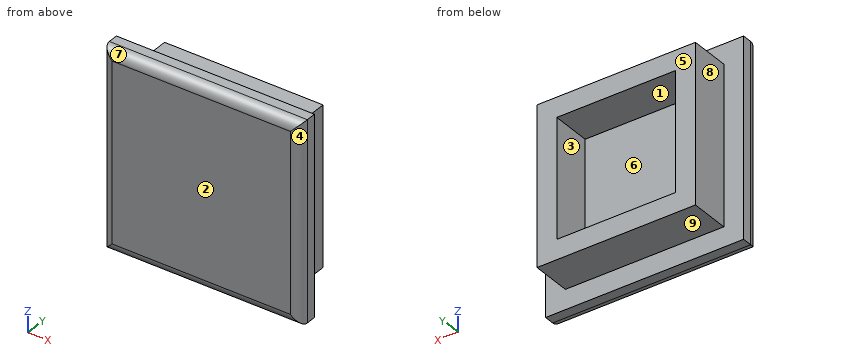
```python
from build123d import *

# Parameters (mm, degrees)
SKETCH1_W           = 20
SKETCH1_H           = 20
BOSS_EXTRUDE1_DEPTH = 2
SKETCH2_W           = 16
SKETCH2_H           = 16
SKETCH2_W_2         = 12
SKETCH2_H_2         = 12
BOSS_EXTRUDE2_DEPTH = 4
FILLET1_R           = 1


with BuildPart() as part:
    # Sketch1 → Boss-Extrude1 (new body)
    with BuildSketch(Plane(origin=(0, 0, 0), x_dir=(1, 0, 0), z_dir=(0, 1, 0))):
        Rectangle(SKETCH1_W, SKETCH1_H)
    extrude(amount=BOSS_EXTRUDE1_DEPTH)

    # Sketch2 → Boss-Extrude2 (add)
    with BuildSketch(Plane(origin=(0, 2, 0), x_dir=(1, 0, 0), z_dir=(0, 1, 0))):
        Rectangle(SKETCH2_W, SKETCH2_H)
        Rectangle(SKETCH2_W_2, SKETCH2_H_2, mode=Mode.SUBTRACT)
    extrude(amount=BOSS_EXTRUDE2_DEPTH)

    # Fillet1
    fillet1_edges = [part.edges().sort_by_distance(p)[0] for p in [
        (0, 0, 10),
        (-10, 0, 0),
        (0, 0, -10),
        (10, 0, 0),
    ]]
    fillet(fillet1_edges, radius=FILLET1_R)


solid = part.part
```
The listing builds one solid part. Answer for the finished solid, in the listing's coordinates (mm). Face numbers are marked on the shaded views. A direction names the side the tool comes from. Coordinates: 2 decimals unless noted, no trailing zeros. Write each loop counter-clockwise with the first axis right and the second up, starting at its lowest first coordinate (ties: lowest second). Pieces come first, ordered by that corner, then holes. Notation, with made-up numbers: (1.5, -9) - (20.5, -9) arc R9 ccw to (20.5, 1) - close; hole circle Ø1 at (78.25, -8.75). An arc over 180 degrees is marked (long way). Return JSON: item names as keys, results as strings. Group by question number.
1. Given pin 1 (3 mm diameter, centred on x = 1, y = 4, fed in from -Z); pin 2 (1.2 mm diameter, centred on y = 3.5, z = 1.5, fed in from -X); pin 3 (2 mm diameter, centred on y = 4.5, z = -5.5, fed in from +X), each flat-ended and moving along its own axis, determine where each tip first touches the part or whether it passes through.
2. A cutting plane is placed at B-B, the plane x = -4.75. Determine the outline of the cut face in (y, z), plus the area to 3 significant figures.
3. Determine the mould class of the marked faces 1, 2, 3 and 4 for opening direction X: released by +X, released by -X, zero draft, split by the parting line, or undercut.
4. Straight lines are drawn through the part: L1, parallel to Z at x = -1, y = 2.9; L2, parallel to Y at x = -4, z = -5.75; L3, parallel to Z at x = 7, y = 2.95. For each, find the intervals that lie inside material, in ascending order.
5. A cutting plane is placed at A-A, the plane z = 1. Determine the outline of the cut face in (x, y).
6. Which of the six approach directions +Z, -Z, +X, -X, +Y, -Y give full straight-line access (tool end or side, diameter ignored) to the marked faces 5, 6, 7, 8 and 9?
7. A cutting plane is placed at D-D, the plane x = -7. Determine the outline of the cut face in (y, z).
8. A cutting plane is placed at C-C, the plane y = 3.4. Determine the outline of the cut face in (x, z).
Ans:
{
 "1": {"pin 1": "z = -8", "pin 2": "x = -8", "pin 3": "x = 8"},
 "2": {"outline": "(0, -9) arc R1 ccw to (1, -10) - (2, -10) - (2, -8) - (6, -8) - (6, -6) - (2, -6) - (2, 6) - (6, 6) - (6, 8) - (2, 8) - (2, 10) - (1, 10) arc R1 ccw to (0, 9) - close", "area": "55.6 mm²"},
 "3": {"face 1": "undercut", "face 2": "zero draft", "face 3": "undercut", "face 4": "released by +X"},
 "4": {"L1": "-8 to -6, 6 to 8", "L2": "0 to 2", "L3": "-8 to 8"},
 "5": {"outline": "(-10, 1) arc R1 ccw to (-9, 0) - (9, 0) arc R1 ccw to (10, 1) - (10, 2) - (8, 2) - (8, 6) - (6, 6) - (6, 2) - (-6, 2) - (-6, 6) - (-8, 6) - (-8, 2) - (-10, 2) - close"},
 "6": {"face 5": "+Z, -Z, +X, -X, +Y", "face 6": "+Y", "face 7": "+Z, +X, -X, -Y", "face 8": "+Z, -Z, -X, +Y", "face 9": "-Z, +X, -X, +Y"},
 "7": {"outline": "(0, -9) arc R1 ccw to (1, -10) - (2, -10) - (2, -8) - (6, -8) - (6, 8) - (2, 8) - (2, 10) - (1, 10) arc R1 ccw to (0, 9) - close"},
 "8": {"outline": "(-8, -8) - (8, -8) - (8, 8) - (-8, 8) - close; hole (-6, -6) - (6, -6) - (6, 6) - (-6, 6) - close"}
}
